Input: part model. Units: mm. Frame: model coordinates. Coordinates: 2 decimals unless noted, no trailing zeros. Loops run counter-clockwise (first coordinate to the right, second up) from the corner with the lowest first, then second, coordinate; pieces in that order, holes last. Notation, with made-up numbers: M 43,28 L 96,28 A16 cw 96,37 Z; hole C 78.5,-27 d9. An arc over 180 degrees is marked long. Use a Markdown table: item, result. Add a question column.
1. Section B-B on y = 3.2. State how many separate pieces and enclosed holes the cut face has, then the cut area to 3 significant figures.
2. Pin query (flat end, axial travel): pin 1 (2.5 mm diameter, centred on x = 0, z = -47.5, fed in from -Y). Return the tip coordinate at first contact, or that it passes through.
3. Line query: L1, parallel to X at y = 1.45, z = 17.5; L2, parallel to X at y = 1.8, z = 44; L3, parallel to Z at x = -4, y = 0.3. Output: solid intervals per line, ascending. Write a range as [from, to].
4. Section A-A on z = 27.5. Output: boundary loops of the cut face in (x, y), then the cut area to 3 significant figures.
Autodesk Inventor part; units mm, degrees
ref_plane "YZ Plane" through (0, 0, 0) normal (1, 0, 0) x (0, 1, 0)
ref_plane "XZ Plane" through (0, 0, 0) normal (0, 1, 0) x (-1, 0, 0)
ref_plane "XY Plane" through (0, 0, 0) normal (0, 0, 1) x (1, 0, 0)
sketch "Sketch1" plane through (0, 0, 0) normal (0, 1, 0) x (-1, 0, 0)
  line L0 (5, 80) -> (-5, 80)
  line L1 (-5, 80) -> (-5, -80)
  line L2 (-5, -80) -> (5, -80)
  line L3 (5, -80) -> (5, 80)
  line L4 (5, 80) -> (-5, -80) construction
  line L5 (-5, 80) -> (5, -80) construction
  point P0 (0, 0)
  dimension "d0" = 10
  dimension "d1" = 160
extrude "Extrusion1" add sketch "Sketch1" along normal blind 4
sketch "Sketch2" plane through (0, 4, 0) normal (0, 1, 0) x (1, 0, 0)
  line L0 (-5, -80) -> (5, -80)
  line L1 (-5, 80) -> (-5, -80)
  line L2 (-5, -80) -> (5, -80)
  line L3 (5, -80) -> (5, 80)
  line L4 (5, 80) -> (-5, 80)
  point P0 (0, 0)
  point P1 (0, -77.5)
  point P2 (0, -72.5)
  point P3 (0, -67.5)
  point P4 (0, -62.5)
  point P5 (0, -57.5)
  point P6 (0, -52.5)
  point P7 (0, -47.5)
  point P8 (0, -42.5)
  point P9 (0, -37.5)
  point P10 (0, -32.5)
  point P11 (0, -27.5)
  point P12 (0, -22.5)
  point P13 (0, -17.5)
  point P14 (0, -12.5)
  point P15 (0, -7.5)
  point P16 (0, -2.5)
  dimension "d4" = 2.5
  dimension "d7" = 5
  dimension "d24" = 0
hole "Hole1" at (0, 4, 77.5) at (0, 4, 72.5) at (0, 4, 67.5) at (0, 4, 62.5) at (0, 4, 57.5) at (0, 4, 52.5) at (0, 4, 47.5) at (0, 4, 42.5) at (0, 4, 37.5) at (0, 4, 32.5) at (0, 4, 27.5) at (0, 4, 22.5) at (0, 4, 17.5) at (0, 4, 12.5) at (0, 4, 7.5) at (0, 4, 2.5) direction (0, -1, 0) diameter 4 end through all
thicken "Thicken1" operation add thickness 1 both sides no extend neighbours yes toward (0, 0, 1) faces at (-1.6667, 1.3333, 80)
thicken "Thicken2" operation add thickness 1 both sides no extend neighbours yes toward (0, 0, -1) faces at (1.6667, 1.3333, -80)
fillet "Fillet1" radius 4 4 edges at (-5, 2, -81) (5, 2, -81) (5, 2, 81) (-5, 2, 81)
mirror "Mirror1" about plane through (0, 0, 0) normal (0, 0, 1) of "Hole1"
properties part number "rearLeg_bot"
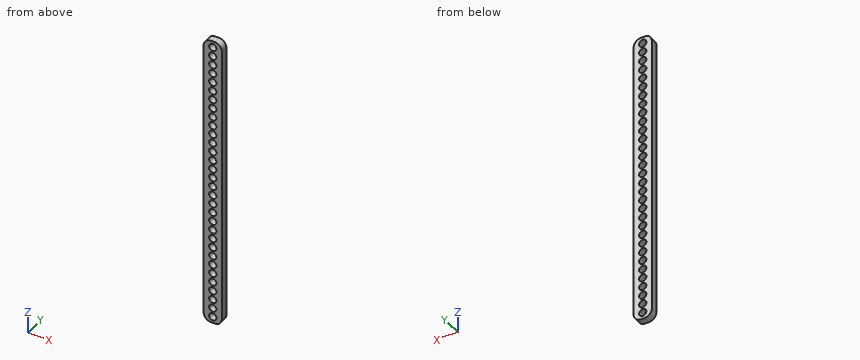
Answers below:
| question | item | result |
|---|---|---|
| 1 | separate pieces | 1 |
| 1 | enclosed holes | 32 |
| 1 | area | 1,200 mm² |
| 2 | pin 1 | passes through |
| 3 | L1 | x = [-5, -2], [2, 5] |
| 3 | L2 | x = [-5, -1.32], [1.32, 5] |
| 3 | L3 | z = [-79.65, 79.65] |
| 4 | outline | M -5,0 L -2,0 L -2,4 L -5,4 Z; M 2,0 L 5,0 L 5,4 L 2,4 Z |
| 4 | area | 24.0 mm² |
